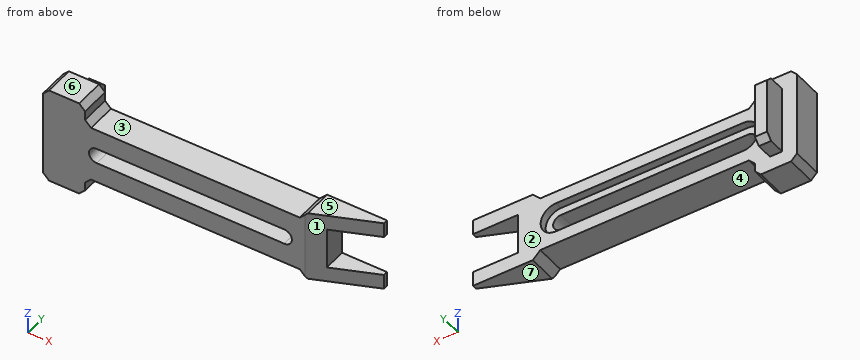
```python
from build123d import *

# Parameters (mm, degrees)
BOSS_EXTRUDE1_DEPTH = 20
CUT_EXTRUDE1_DEPTH  = 5
CUT_EXTRUDE2_DEPTH  = 132.297386022
CHAMFER1_SIZE       = 4
BOSS_EXTRUDE2_DEPTH = 15
CHAMFER2_SIZE       = 4
BOSS_EXTRUDE3_DEPTH = 20
CHAMFER3_SIZE       = 5
CUT_EXTRUDE3_DEPTH  = 60
SCALE2_SCALE        = 0.19


with BuildPart() as part:
    # Sketch1 → Boss-Extrude1 (new body)
    with BuildSketch(Plane(origin=(0, 0, 0), x_dir=(1, 0, 0), z_dir=(0, 1, 0))):
        Polygon((-26.074130493, -28.215811716), (-26.074130493, -42.310360901), (-54.263228862, -42.310360901), (-54.263228862, 23.128617456), (-26.074130493, 23.128617456), (-26.074130493, 9.28575665), (122.67370108, 9.28575665), (122.67370108, -28.215811716), align=None)
    extrude(amount=BOSS_EXTRUDE1_DEPTH)

    # Sketch2 → Cut-Extrude1 (cut)
    with BuildSketch(Plane(origin=(0, 20, 0), x_dir=(1, 0, 0), z_dir=(0, 1, 0))):
        with BuildLine():
            Line((-18.280512059, 0.584936596), (107.256828457, 0.584936596))
            ThreePointArc((107.256828457, 0.584936596), (117.432636776, -9.590871723), (107.256828457, -19.766680041))
            Line((107.256828457, -19.766680041), (-18.280512059, -19.766680041))
            ThreePointArc((-18.280512059, -19.766680041), (-28.456320377, -9.590871723), (-18.280512059, 0.584936596))
        make_face()
        with BuildLine():
            Line((-18.280512059, -4.415063404), (107.256828457, -4.415063404))
            ThreePointArc((107.256828457, -4.415063404), (112.432636776, -9.590871723), (107.256828457, -14.766680041))
            Line((107.256828457, -14.766680041), (-18.280512059, -14.766680041))
            ThreePointArc((-18.280512059, -14.766680041), (-23.456320377, -9.590871723), (-18.280512059, -4.415063404))
        make_face(mode=Mode.SUBTRACT)
    extrude(amount=-CUT_EXTRUDE1_DEPTH, mode=Mode.SUBTRACT)

    # Sketch3 → Cut-Extrude2 (cut, through all)
    with BuildSketch(Plane(origin=(0, 20, 0), x_dir=(1, 0, 0), z_dir=(0, 1, 0))):
        with BuildLine():
            Line((-18.280512059, -14.766680041), (107.256828457, -14.766680041))
            ThreePointArc((107.256828457, -14.766680041), (112.432636776, -9.590871723), (107.256828457, -4.415063404))
            Line((107.256828457, -4.415063404), (-18.280512059, -4.415063404))
            ThreePointArc((-18.280512059, -4.415063404), (-23.456320377, -9.590871723), (-18.280512059, -14.766680041))
        make_face()
    extrude(amount=-CUT_EXTRUDE2_DEPTH, mode=Mode.SUBTRACT)

    # Chamfer1
    chamfer1_edges = [part.edges().sort_by_distance(p)[0] for p in [
        (-26.074130493, 10, 28.215811716),
        (-26.074130493, 10, -9.28575665),
        (-26.074130493, 10, -23.128617456),
        (-54.263228862, 10, -23.128617456),
        (-54.263228862, 10, 42.310360901),
        (-26.074130493, 10, 42.310360901),
    ]]
    chamfer(chamfer1_edges, length=CHAMFER1_SIZE)

    # Sketch4 → Boss-Extrude2 (add)
    with BuildSketch(Plane(origin=(0, 20, 0), x_dir=(1, 0, 0), z_dir=(0, 1, 0))):
        Polygon((-36.074130493, -32.215811716), (-36.074130493, 13.128617456), (-44.263228862, 13.128617456), (-44.263228862, -32.310360901), (-36.074130493, -32.310360901), align=None)
    extrude(amount=BOSS_EXTRUDE2_DEPTH)

    # Chamfer2
    chamfer2_edges = [part.edges().sort_by_distance(p)[0] for p in [
        (-40.168679677, 35, -13.128617456),
        (-40.168679677, 35, 32.310360901),
    ]]
    chamfer(chamfer2_edges, length=CHAMFER2_SIZE)

    # Sketch5 → Boss-Extrude3 (add)
    with BuildSketch(Plane(origin=(0, 20, 0), x_dir=(1, 0, 0), z_dir=(0, 1, 0))):
        Polygon((122.67370108, -33.215811716), (162.735602204, -33.215811716), (162.735602204, -23.215811716), (132.67370108, -23.215811716), (132.67370108, 4.28575665), (162.735602204, 4.28575665), (162.735602204, 14.28575665), (122.67370108, 14.28575665), align=None)
    extrude(amount=-BOSS_EXTRUDE3_DEPTH)

    # Chamfer3
    chamfer3_edges = [part.edges().sort_by_distance(p)[0] for p in [
        (122.67370108, 10, -9.28575665),
        (122.67370108, 10, 28.215811716),
    ]]
    chamfer(chamfer3_edges, length=CHAMFER3_SIZE - 0.0001)  # a hair under: the kernel refuses the full size

    # Sketch6 → Cut-Extrude3 (cut)
    with BuildSketch(Plane.XY.offset(33.215811716)):
        Polygon((120.800441338, -0.153311602), (162.735602204, 16.953910153), (162.735602204, 0), align=None)
    extrude(amount=-CUT_EXTRUDE3_DEPTH, mode=Mode.SUBTRACT)


with BuildPart() as part_1:
    # Scale2: scaled about (30.500255958, 10.567938769, 9.471238373)
    add(part.part.scale(SCALE2_SCALE).moved(Location((24.705207326, 8.560030403, 7.671703082))))


solid = part_1.part
```
CAD build for the part. Positions are in the model's coordinates, mm. Face numbers are marked on the shaded views. A direction names the side the tool comes from. Coordinates: 2 decimals unless noted, no trailing zeros. Write each loop counter-clockwise with the first axis right and the second up, starting at its lowest first coordinate (ties: lowest second). Pieces come first, ordered by that corner, then holes.
(1) Cut at C-C, the plane z = 9.5. List the corners of the cut face in (x, y).
(2) Cut at A-A, the plane x = 36.5. List the corners of the cut face in (y, z).
(3) Drill centre lines: probe 1 along Z at (x, y) = (53, 11); probe 2 along Z at (x, y) = (23.5, 9.75); probe 3 along X at (y, z) = (14, 9.75). Where is each one in solid material? Low to high.
(4) 3-axis set-ups, long thin cutter, end or side, ignore diameter. For the marked faces 4, 5, 6 and 7: which of +Z, -Z, +X, -X, +Y, -Y reach the whole face in a straight line?
(5) Two-plate mould, pull along X, no slides. Class the marked faces 1, 2 and 3: +X half, -X half, draft (parallel to the pull), parting line (faces both ways), or undercut.
(6) Flat gauge pins, fed straight in: pin 1 (2.5 mm diameter, centred on y = 13.5, z = 10, fed in from +X); pin 2 (0.9 mm diameter, centred on x = 52.5, y = 11, fed in from -Z); pin 3 (4 mm diameter, centred on x = 22.5, z = 5, fed in from +Y); pin 4 (1.4 mm diameter, centred on y = 13, z = 11.5, fed in from -X). Where does each tip first touch, or does it go through?
(7) Cut at D-D, the plane z = 4.5. List the corners of the cut face in (x, y).
Geometry says:
1. outline: (14.4, 8.56) - (20.25, 8.56) - (20.25, 11.41) - (19.3, 11.41) - (19.3, 12.36) - (17.85, 12.36) - (17.85, 15.21) - (16.3, 15.21) - (16.3, 12.36) - (14.4, 12.36) - close; (46.07, 8.56) - (47.73, 8.56) - (49.91, 9.45) - (49.91, 12.36) - (47.02, 12.36) - (47.02, 11.41) - (46.07, 11.41) - close
2. outline: (8.56, 5.91) - (12.36, 5.91) - (12.36, 7.56) - (11.41, 7.56) - (11.41, 8.51) - (8.56, 8.51) - close; (8.56, 10.48) - (11.41, 10.48) - (11.41, 11.43) - (12.36, 11.43) - (12.36, 13.03) - (8.56, 13.03) - close
3. probe 1: z = 4.96 to 6.86, 12.08 to 13.98
3. probe 2: z = 5.91 to 8.51, 10.48 to 13.03
3. probe 3: x = 16.3 to 17.85
4. face 4: -Z, +Y, -Y
4. face 5: +Z, +X, +Y, -Y
4. face 6: +Z, +X, -X, +Y, -Y
4. face 7: -Z, +X, +Y, -Y
5. face 1: +X half
5. face 2: draft
5. face 3: undercut
6. pin 1: stops at x = 49.91
6. pin 2: stops at z = 4.96
6. pin 3: stops at y = 12.36
6. pin 4: stops at x = 14.4
7. outline: (14.4, 8.56) - (19.75, 8.56) - (19.75, 12.36) - (14.4, 12.36) - close
